Build history of the part. All positions in model axes, mm. A direction names the side the tool comes from. Give positions to 0.01 mm unless a question says otherwise; leave off trailing zeros. Loops run counter-clockwise (first coordinate to the right, second up) from the corner with the lowest first, then second, coordinate; pieces in that order, holes last. Notation, with made-up numbers: (73.25, 80.25) -> (112.25, 80.25) arc R13 cw to (112.25, 88.25) -> close; hole circle Ø11 at (58.25, 45). An arc over 180 degrees is marked (long way). One line per question, with ' | ' between items. Start each with the question number.
(1) Drill centre lines: L1, parallel to Y at x = -0.1, z = 0.95; L2, parallel to Z at x = 1.4, y = -2; L3, parallel to X at y = -0.25, z = 2.25. Where is each one in solid material? Low to high. Write a range as from..to.
(2) Flat gauge pins, fed straight in: pin 1 Ø3 at (x, y) = (-1.5, 2.5) entering from +Z; pin 2 Ø3 at (x, y) = (-1, 2.5) entering from +Z; pin 3 Ø3 at (x, y) = (-1, -1.5) entering from +Z. Where does each tip first touch, or does it go through?
(3) Mould opens along Y. For faces 1 (the face through (-1.3, -1.4, 0)), 2 (the face through (1.394, -2.37, 1.479)), 3 (the face through (0, 0, 3)) say: pulls with the +Y half, pulls with the -Y half, needs draft (parallel to the pull), parting line crosses it, or undercut.
(4) 3-axis set-ups, long thin cutter, end or side, ignore diameter. For faces 4 (the face through (2.75, 0, 1)), 5 (the face through (-1.5, -0.07, 1.48)): which of +Z, -Z, +X, -X, +Y, -Y reach the whole face in a straight line?
(5) Slice it at B-B, the plane y = 2.5. Write the cut outline in (x, z).
(6) Slice it at A-A, the plane z = 1.6. Write the cut outline in (x, y).
Autodesk Inventor part; units mm, degrees
ref_plane "YZ Plane" through (0, 0, 0) normal (1, 0, 0) x (0, 1, 0)
ref_plane "XZ Plane" through (0, 0, 0) normal (0, 1, 0) x (-1, 0, 0)
ref_plane "XY Plane" through (0, 0, 0) normal (0, 0, 1) x (1, 0, 0)
sketch "Sketch1" plane through (0, 0, 0) normal (0, 0, 1) x (1, 0, 0)
  line L0 (2.75, 1.5877) -> (2.75, -1.5877)
  line L1 (2.75, -1.5877) -> (0, -3.1754)
  line L2 (0, -3.1754) -> (-2.75, -1.5877)
  line L3 (-2.75, -1.5877) -> (-2.75, 1.5877)
  line L4 (-2.75, 1.5877) -> (0, 3.1754)
  line L5 (0, 3.1754) -> (2.75, 1.5877)
  circle A0 centre (0, 0) radius 1.5
  dimension "d0" = 5.5
  dimension "d1" = 3
extrude "Extrusion1" add sketch "Sketch1" along normal blind 3
sketch "Sketch2" plane through (0, 0, 0) normal (1, 0, 0) x (0, 1, 0)
  line L0 (2.3816, 3) -> (2.3816, 4.1867) construction
  line L1 (2.3816, 4.1867) -> (0, 6.751) construction
  line L2 (0, 6.751) -> (-2.3816, 4.1867) construction
  line L3 (-2.3816, 4.1867) -> (-2.3816, 3) construction
  spline S0 degree 4 poles (2.3816, 3) (2.3816, 4.1867) (0, 6.751) (-2.3816, 4.1867) (-2.3816, 3) knots 1 1 1 1 1 2 2 2 2 2
  line L4 (0.553, 5) -> (-1.6263, 5)
  line L5 (-3.1754, 0) -> (-1.5877, 0)
  line L6 (-1.5877, 3) -> (1.5877, 3)
  line L7 (-3.1754, 3) -> (-1.5877, 3)
  line L8 (1.5877, 3) -> (3.1754, 3)
  line L9 (2.3816, 3) -> (-2.3816, 3)
  line L10 (0, 3) -> (0, 6.751)
  line L11 (1.5877, 3) -> (-1.5877, 3)
  point P0 (0, 0)
  point P1 (0, 5)
  dimension "d4" = 5
revolve "Revolution1" add sketch "Sketch2" angle 360 about axis through (0, 0, 3) along (0, 0, 1) contours L8 L6 L10 S0
thread "Thread1"
properties part number "M3 Acorn Nut"
Final values:
1) L1: -3.12..-1.5, 1.5..3.12 | L2: 0..3 | L3: -2.75..-1.48, 1.48..2.75
2) pin 1: z = 4.53 | pin 2: z = 4.67 | pin 3: z = 4.98
3) face 1: needs draft | face 2: pulls with the -Y half | face 3: undercut
4) face 4: +Z, -Z, +X, +Y, -Y | face 5: -Z
5) outline: (-1.17, 0) -> (1.17, 0) -> (1.17, 3) -> (-1.17, 3) -> close
6) outline: (-2.75, -1.59) -> (0, -3.18) -> (2.75, -1.59) -> (2.75, 1.59) -> (0, 3.18) -> (-2.75, 1.59) -> close; hole circle Ø3 at (0, 0)
